Geometry check sheet. Reference: the model listing, model coordinates, mm. Face numbers are marked on the shaded views. A direction names the side the tool comes from. Coordinates: 2 decimals unless noted, no trailing zeros. Write each loop counter-clockwise with the first axis right and the second up, starting at its lowest first coordinate (ties: lowest second). Pieces come first, ordered by that corner, then holes. Notation, with made-up numbers: (54, 44.5) -> (113, 44.5) arc R9 cw to (113, 48.5) -> close; hole circle Ø7 at (-21.75, 86.25). An arc over 180 degrees is marked (long way). Answer in a Markdown table with one row per item. Add a question column.
Q1. Section check A-A, the plane z = -11.75. Record the boundary of the cut face in (x, y).
Q2. Thickness scan on line 1 (Z direction, x = 2.25, y = -1.75); line 2 (Y direction, x = -1, z = -6.5); line 3 (X direction, y = 2.5, z = 2). Record the ranges inside material, lowest first.
Q3. Tool access check on the marked faces 1 and 2. Record the directions out of +Z, -Z, +X, -X, +Y, -Y that give a thin tool (end or side, any length) a straight path to the whole face; none if there is none.
Q4. Gauge pin test, flat ends, axial feed: P1, Ø2, axis at y = 2.5, z = 0.5, coming from the +X side; P2, Ø1, axis at x = 0, y = 0.5, coming from the +Z side; P3, Ø3, axis at x = -1.5, z = -2.5, coming from the -Y side. Record the tip position at first contact, or that the pin passes through.
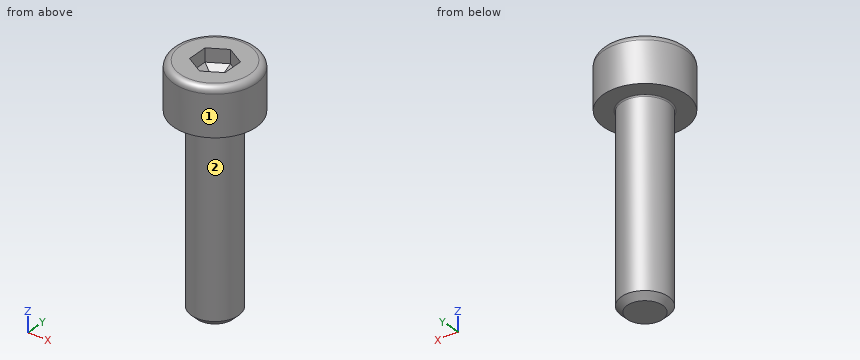
```python
from build123d import *
from OCP.BRepFilletAPI import BRepFilletAPI_MakeChamfer

# Parameters (mm, degrees)
SKETCH_1_R          = 3.5
EXTRUDE_1_DEPTH     = 4
CUT_EXTRUDE_1_DEPTH = 2
SKETCH_3_R          = 2
EXTRUDE_2_DEPTH     = 16
CHAMFER_1_SIZE      = 0.5
FILLET_1_R          = 0.538461538
CHAMFER_2_SIZE      = 0.864553314
CHAMFER_2_SIZE2     = 1.497450266
FILLET_2_R          = 0.1


with BuildPart() as part:
    # Sketch 1 → Extrude 1 (new body)
    with BuildSketch(Plane.XY):
        Circle(SKETCH_1_R)
    extrude(amount=EXTRUDE_1_DEPTH)

    # Sketch 2 → Cut-Extrude 1 (cut)
    with BuildSketch(Plane.XY.offset(4)):
        Polygon((1.5, 0.866025404), (0, 1.732050808), (-1.5, 0.866025404), (-1.5, -0.866025404), (0, -1.732050808), (1.5, -0.866025404), align=None)
    extrude(amount=-CUT_EXTRUDE_1_DEPTH, mode=Mode.SUBTRACT)

    # Sketch 3 → Extrude 2 (add)
    with BuildSketch(Plane(origin=(0, 0, 0), x_dir=(-1, 0, 0), z_dir=(0, 0, -1))):
        with Locations(Location((0, 0, 0), (0, 0, 180))):
            Circle(SKETCH_3_R)
    extrude(amount=EXTRUDE_2_DEPTH)

    # Chamfer 1
    chamfer_1_edges = [part.edges().sort_by_distance(p)[0] for p in [
        (-2, 0, -16),
    ]]
    chamfer(chamfer_1_edges, length=CHAMFER_1_SIZE)

    # Fillet 1
    fillet_1_edges = [part.edges().sort_by_distance(p)[0] for p in [
        (-3.5, 0, 4),
    ]]
    fillet(fillet_1_edges, radius=FILLET_1_R)

    # Chamfer 2: one chamfer whose edges measure the first distance from different faces: ONE call of the kernel's chamfer builder (chamfer() names one face for all edges)
    chamfer_2_edges_1 = [part.edges().sort_by_distance(p)[0] for p in [
        (-0.75, 1.299038106, 2),
    ]]
    chamfer_2_side_1 = [part.faces().sort_by_distance(p)[0] for p in [
        (-0.75, 1.299038106, 3),
    ]]
    chamfer_2_edges_2 = [part.edges().sort_by_distance(p)[0] for p in [
        (0.75, 1.299038106, 2),
    ]]
    chamfer_2_side_2 = [part.faces().sort_by_distance(p)[0] for p in [
        (0.75, 1.299038106, 3),
    ]]
    chamfer_2_edges_3 = [part.edges().sort_by_distance(p)[0] for p in [
        (1.5, 0, 2),
    ]]
    chamfer_2_side_3 = [part.faces().sort_by_distance(p)[0] for p in [
        (1.5, 0, 3),
    ]]
    chamfer_2_edges_4 = [part.edges().sort_by_distance(p)[0] for p in [
        (0.75, -1.299038106, 2),
    ]]
    chamfer_2_side_4 = [part.faces().sort_by_distance(p)[0] for p in [
        (0.75, -1.299038106, 3),
    ]]
    chamfer_2_edges_5 = [part.edges().sort_by_distance(p)[0] for p in [
        (-0.75, -1.299038106, 2),
    ]]
    chamfer_2_side_5 = [part.faces().sort_by_distance(p)[0] for p in [
        (-0.75, -1.299038106, 3),
    ]]
    chamfer_2_edges_6 = [part.edges().sort_by_distance(p)[0] for p in [
        (-1.5, 0, 2),
    ]]
    chamfer_2_side_6 = [part.faces().sort_by_distance(p)[0] for p in [
        (-1.5, 0, 3),
    ]]
    chamfer_2 = BRepFilletAPI_MakeChamfer(part.part.solid().wrapped)
    for e in chamfer_2_edges_1:
        chamfer_2.Add(CHAMFER_2_SIZE, CHAMFER_2_SIZE2, e.wrapped, chamfer_2_side_1[0].wrapped)  # the first distance lies on this face
    for e in chamfer_2_edges_2:
        chamfer_2.Add(CHAMFER_2_SIZE, CHAMFER_2_SIZE2, e.wrapped, chamfer_2_side_2[0].wrapped)  # the first distance lies on this face
    for e in chamfer_2_edges_3:
        chamfer_2.Add(CHAMFER_2_SIZE, CHAMFER_2_SIZE2, e.wrapped, chamfer_2_side_3[0].wrapped)  # the first distance lies on this face
    for e in chamfer_2_edges_4:
        chamfer_2.Add(CHAMFER_2_SIZE, CHAMFER_2_SIZE2, e.wrapped, chamfer_2_side_4[0].wrapped)  # the first distance lies on this face
    for e in chamfer_2_edges_5:
        chamfer_2.Add(CHAMFER_2_SIZE, CHAMFER_2_SIZE2, e.wrapped, chamfer_2_side_5[0].wrapped)  # the first distance lies on this face
    for e in chamfer_2_edges_6:
        chamfer_2.Add(CHAMFER_2_SIZE, CHAMFER_2_SIZE2, e.wrapped, chamfer_2_side_6[0].wrapped)  # the first distance lies on this face
    add(Compound.cast(chamfer_2.Shape()), mode=Mode.REPLACE)

    # Fillet 2
    fillet_2_edges = [part.edges().sort_by_distance(p)[0] for p in [
        (-2, 0, 0),
    ]]
    fillet(fillet_2_edges, radius=FILLET_2_R)


solid = part.part
```
Calculated:
| question | item | result |
|---|---|---|
| 1 | outline | circle Ø4 at (0, 0) |
| 2 | line 1 | z = 0 to 4 |
| 2 | line 2 | y = -1.73 to 1.73 |
| 2 | line 3 | x = -2.45 to 2.45 |
| 3 | face 1 | +Z, -Z |
| 3 | face 2 | -Z |
| 4 | P1 | stops at x = 3.16 |
| 4 | P2 | stops at z = 2.54 |
| 4 | P3 | stops at y = -2 |
